from build123d import *

# Parameters (mm, degrees)
F0_R     = 75
F0_R_2   = 25
F1_DEPTH = 28
F2_R     = 48.1474701807
F2_R_2   = 25
F3_DEPTH = 9
F4_R     = 39.9409386185
F4_R_2   = 25
F5_DEPTH = 15


with BuildPart() as f1:
    # F0 (on Top) → F1 (new body)
    with BuildSketch(Plane.XY):
        Circle(F0_R)
        Circle(F0_R_2, mode=Mode.SUBTRACT)
    extrude(amount=F1_DEPTH)

    # F2 (on face) → F3 (join)
    with BuildSketch(Plane.XY.offset(28)):
        Circle(F2_R)
        Circle(F2_R_2, mode=Mode.SUBTRACT)
    extrude(amount=F3_DEPTH)

    # F4 (on face) → F5 (join)
    with BuildSketch(Plane.XY.offset(37)):
        Circle(F4_R)
        Circle(F4_R_2, mode=Mode.SUBTRACT)
    extrude(amount=-F5_DEPTH)


solid = f1.part
Source: CAD feature listing. Evaluate the final solid. Frame: model axes, mm. A direction names the side the tool comes from. Round coordinates to 2 decimals unless told otherwise and drop trailing zeros. Loops run counter-clockwise (first coordinate to the right, second up) from the corner with the lowest first, then second, coordinate; pieces in that order, holes last.
Q1. First-contact query: P1, Ø10, axis at y = -14.5, z = 10.5, coming from the -X side; P2, Ø1.5, axis at x = 51.5, z = 6, coming from the +Y side; P3, Ø6, axis at x = 44.5, z = 11, coming from the +Y side; P4, Ø5, axis at x = 21.5, y = -37, coming from the -Z side. Flat tips, straight axial feed; report the tip coordinate or a pass-through.
Q2. Section D-D, the plane x = -42. Return loops of the section in (y, z), plus the area to 3 significant figures.
Q3. Ray query, line 1 (Y direction, x = 0, z = 21); line 2 (Z direction, x = 58.5, y = -33.5); line 3 (X direction, y = 3.5, z = 19). Return the intervals inside material, ascending.
Q4. Section A-A, the plane y = 0. Return loops of the section in (x, z), plus the area to 3 significant figures.
Q5. Access query for faces 4 (the face through (21, -21, 37)), 5 (the face through (45.924, 14.462, 32.437)). Directions: +Z, -Z, +X, -X, +Y, -Y. A direction counts if a zero-diameter tool reaches every point of the face in a straight line with its end or side. Return the directions, or none.
Q6. Section C-C, the plane z = 34.5. Return loops of the section in (x, y), plus the area to 3 significant figures.
Q7. Mould query, pull axis Y, two halves, no side actions, for faces 1 (the face through (-9.764, 74.362, 13.804)), 2 (the face through (23.846, 7.509, 18.241)), 3 (the face through (-1, -49, 28)). Classes: pulls with the +Y half, pulls with the -Y half, needs draft (parallel to the pull), parting line crosses it, or undercut.
Solutions:
1. P1: stops at x = -74.4
1. P2: stops at y = 55.22
1. P3: stops at y = 62.47
1. P4: stops at z = 0
2. outline: (-62.14, 0) - (62.14, 0) - (62.14, 28) - (23.54, 28) - (23.54, 37) - (-23.54, 37) - (-23.54, 28) - (-62.14, 28) - close
2. area: 3,900 mm2
3. line 1: y = -75 to -25, 25 to 75
3. line 2: z = 0 to 28
3. line 3: x = -74.92 to -24.75, 24.75 to 74.92
4. outline: (-75, 0) - (-25, 0) - (-25, 37) - (-48.15, 37) - (-48.15, 28) - (-75, 28) - close; (25, 0) - (75, 0) - (75, 28) - (48.15, 28) - (48.15, 37) - (25, 37) - close
4. area: 3,220 mm2
5. face 4: +Z, +X, -X, +Y, -Y
5. face 5: +Z
6. outline: circle Ø96.29 at (0, 0); hole circle Ø50 at (0, 0)
6. area: 5,320 mm2
7. face 1: parting line crosses it
7. face 2: undercut
7. face 3: needs draft
